The figure shows three views and two pictorial views of one solid part (mm, origin at its lowest corner). Answer the questions. Coordinates: 2 decimals unless noted, no trailing zeros. Loops run counter-clockwise (first coordinate to the right, second up) from the corner with the lowest first, then second, coordinate; pieces in that order, holes last.
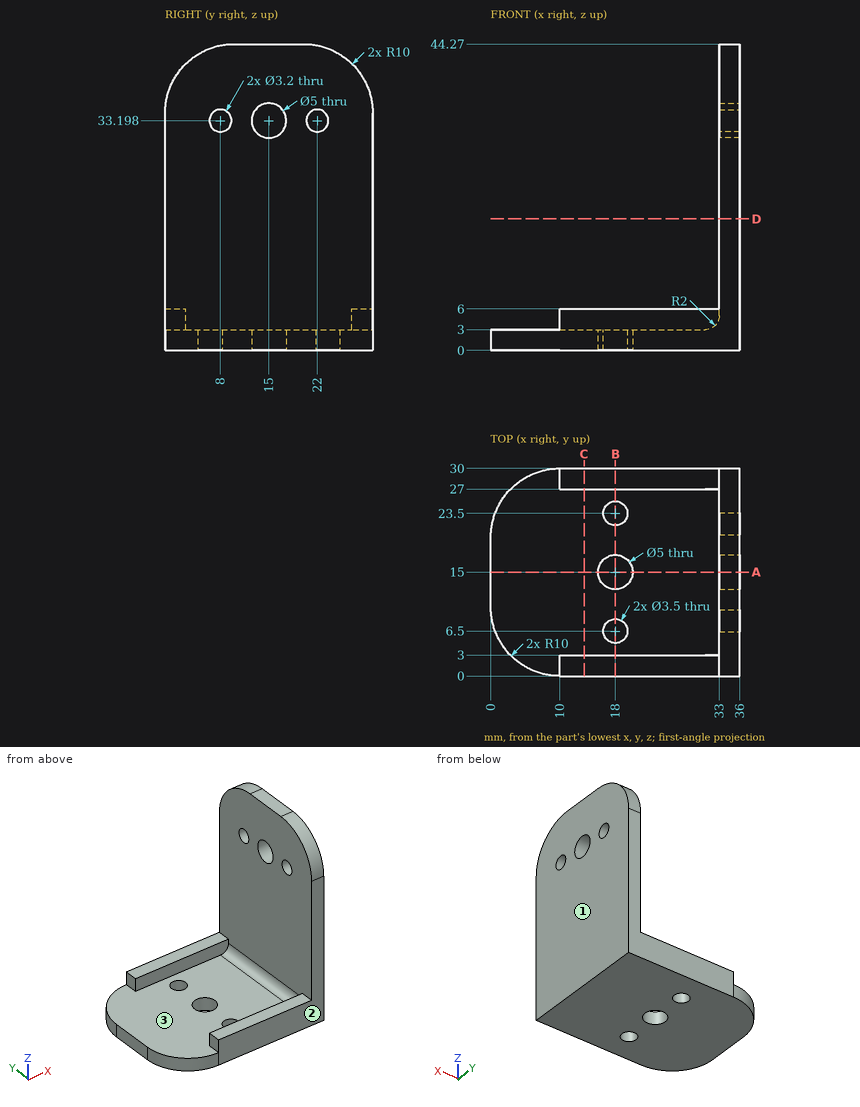
Q1. Straight lines are drawn through the part: probe 1 along Y at (x, z) = (18, 1.7); probe 2 along Z at (x, y) = (9, 21.25); probe 3 along X at (y, z) = (9, 39). For each, find the intervals that lie inside material, in ascending order.
Findings below:
probe 1: y = 0 to 4.75, 8.25 to 12.5, 17.5 to 21.75, 25.25 to 30
probe 2: z = 0 to 3
probe 3: x = 33 to 36
Q2. A cutting plane is placed at D-D (z = 19). Give the vertices of the cut face in (x, y).
Findings below:
outline: (33, 0) - (36, 0) - (36, 30) - (33, 30) - close
Q3. A cutting plane is placed at B-B (x = 18). Give the vertices of the cut face in (y, z).
Findings below:
outline: (0, 0) - (4.75, 0) - (4.75, 3) - (3, 3) - (3, 6) - (0, 6) - close; (8.25, 0) - (12.5, 0) - (12.5, 3) - (8.25, 3) - close; (17.5, 0) - (21.75, 0) - (21.75, 3) - (17.5, 3) - close; (25.25, 0) - (30, 0) - (30, 6) - (27, 6) - (27, 3) - (25.25, 3) - close
Q4. Flat-ended cylindrical pins translate along their axes: pin 1 Ø10 at (x, y) = (6, 10) entering from +Z; pin 2 Ø1.5 at (x, y) = (18, 29) entering from +Z; pin 3 Ø4 at (x, y) = (18, 15) entering from +Z; pin 4 Ø9 at (y, z) = (12.5, 30) entering from -X. Find the tip coordinate at first contact, or state that the pin passes through.
Findings below:
pin 1: stops at z = 3
pin 2: stops at z = 6
pin 3: passes through
pin 4: stops at x = 33
Q5. A cutting plane is placed at C-C (x = 13.5). Give the vertices of the cut face in (y, z), then the cut area to 3 significant figures.
Findings below:
outline: (0, 0) - (30, 0) - (30, 6) - (27, 6) - (27, 3) - (3, 3) - (3, 6) - (0, 6) - close
area: 108 mm2
Q6. Determine the mould class of the marked faces 1, 2 and 3 for opening direction Y: +Y half, -Y half, draft (parallel to the pull), parting line (faces both ways), or undercut.
Findings below:
face 1: draft
face 2: -Y half
face 3: undercut
Q7. A cutting plane is placed at A-A (y = 15). Give the vertices of the cut face in (x, z), then the cut area to 3 significant figures.
Findings below:
outline: (0, 0) - (15.5, 0) - (15.5, 3) - (0, 3) - close; (20.5, 0) - (36, 0) - (36, 30.7) - (33, 30.7) - (33, 5) arc R2 cw to (31, 3) - (20.5, 3) - close; (33, 35.7) - (36, 35.7) - (36, 44.27) - (33, 44.27) - close
area: 203 mm2
